Check sheet for the modelled part. Datum: model origin and axes. Units: mm. Face numbers are marked on the shaded views. A direction names the side the tool comes from. Round coordinates to 2 decimals unless told otherwise and drop trailing zeros. Loops run counter-clockwise (first coordinate to the right, second up) from the corner with the lowest first, then second, coordinate; pieces in that order, holes last. Notation, with made-up numbers: (51.5, 44.5) - (91.5, 44.5) arc R28 cw to (91.5, 73.5) - close; hole circle Ø8 at (29.5, 81.25). An arc over 180 degrees is marked (long way). Answer in a Markdown table with one row per item. Add a question column.
(1) Cross-section at D-D on y = 9.25. Enter the section's corners in (x, z) (3 decimals), then the cut area to 3 significant figures.
(2) Cross-section at B-B on x = 22. Enter the section's corners in (y, z), then the cut area to 3 significant figures.
(3) Thickness scan on line 1 along X through (y, z) = (-10, 9.5); line 2 along X through (y, z) = (6, 4); line 3 along Z through (x, y) = (25.4, 1.5) (3 decimals). Record the ranges inside material, lowest first.
(4) Access from +Z, -Z, +X, -X, +Y, -Y to the whole of each face (thin tool, end or side, straight path). Record for the marked faces 4, 5, 6, 7 and 8.
(5) Gauge pin test, flat ends, axial feed: pin 1 (1.1 mm diameter, centred on x = 14, y = 1, fed in from -Z); pin 2 (2 mm diameter, centred on y = 5, z = 18, fed in from +X); pin 3 (2 mm diameter, centred on x = 21, y = 4, fed in from +Z); pin 4 (7.5 mm diameter, centred on x = 25.4, z = 9.525, fed in from -Y). Record the tip position at first contact, or that the pin passes through.
(6) Cross-section at C-C on y = 3.75. Enter the section's corners in (x, z) (3 decimals).
(7) Mould release check, pull along X, two halves, no side actions. Record for the marked faces 1, 2 and 3: +X half, -X half, draft (parallel to the pull), parting line (faces both ways), or undercut.
(8) Cross-section at A-A on z = 7.5. Enter the section's corners in (x, y), then the cut area to 3 significant figures.
from build123d import *

# Parameters (mm, degrees)
F0_W     = 12.7
F0_H     = 25.4
F1_DEPTH = 12.7
F3_DEPTH = 12.7
F4_W     = 12.7
F4_H     = 12.7
F5_DEPTH = 12.7
F6_R     = 9.525
F7_DEPTH = 12.7
F8_R     = 6.35
F9_DEPTH = 25.4


with BuildPart() as f1:
    # F0 (on Front) → F1 (new body, symmetric)
    with BuildSketch(Plane.XZ):
        with Locations((6.35, 12.7)):
            Rectangle(F0_W, F0_H)
    extrude(amount=F1_DEPTH, both=True)

    # F2 (on face) → F3 (cut)
    with BuildSketch(Plane.YZ.offset(12.7)):
        Polygon((-12.7, 25.4), (-12.7, 19.05), (-6.35, 25.4), align=None)
        Polygon((12.7, 25.4), (6.35, 25.4), (12.7, 19.05), align=None)
    extrude(amount=-F3_DEPTH, mode=Mode.SUBTRACT)

    # F4 (on face) → F5 (join)
    with BuildSketch(Plane.YZ.offset(12.7)):
        with Locations((0, 12.7)):
            Rectangle(F4_W, F4_H)
    extrude(amount=F5_DEPTH)

    # F6 (on Front) → F7 (join, symmetric)
    with BuildSketch(Plane.XZ):
        with Locations((25.4, 9.525)):
            Circle(F6_R)
    extrude(amount=F7_DEPTH, both=True)

    # F8 (on face) → F9 (cut)
    with BuildSketch(Plane.XZ.offset(12.7)):
        with Locations((25.4, 9.525)):
            Circle(F8_R)
    extrude(amount=-F9_DEPTH, mode=Mode.SUBTRACT)


solid = f1.part
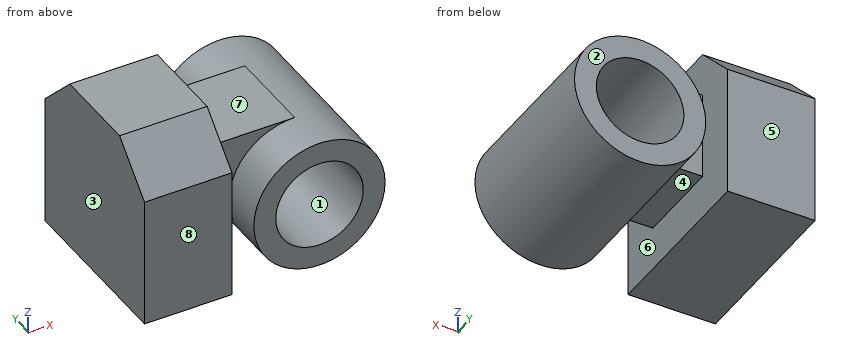
Answers:
| question | item | result |
|---|---|---|
| 1 | outline | (0, 0) - (12.7, 0) - (12.7, 22.5) - (0, 22.5) - close; circle Ø19.05 at (25.4, 9.525); hole circle Ø12.7 at (25.4, 9.525) |
| 1 | area | 444 mm^2 |
| 2 | outline | (-12.7, 0.63) - (12.7, 0.63) - (12.7, 4.16) - (-12.7, 4.16) - close; (-12.7, 14.89) - (12.7, 14.89) - (12.7, 18.42) - (6.35, 18.42) - (6.35, 19.05) - (-6.35, 19.05) - (-6.35, 18.42) - (-12.7, 18.42) - close |
| 2 | area | 188 mm^2 |
| 3 | line 1 | x = 0 to 12.7, 15.88 to 19.05, 31.75 to 34.92 |
| 3 | line 2 | x = 0 to 12.7, 17.64 to 22.27, 28.53 to 33.16 |
| 3 | line 3 | z = 0 to 3.175, 15.875 to 19.05 |
| 4 | face 4 | -Z, +Y, -Y |
| 4 | face 5 | +Z, -Z, +X, -X, +Y |
| 4 | face 6 | none |
| 4 | face 7 | +Z, +X, +Y, -Y |
| 4 | face 8 | +Z, -Z, +X, -X, -Y |
| 5 | pin 1 | stops at z = 6.35 |
| 5 | pin 2 | stops at x = 31.3 |
| 5 | pin 3 | stops at z = 19.05 |
| 5 | pin 4 | passes through |
| 6 | outline | (0, 0) - (12.7, 0) - (12.7, 6.35) - (16.42, 6.35) arc R9.525 ccw (long way) to (25.4, 19.05) - (12.7, 19.05) - (12.7, 25.4) - (0, 25.4) - close; hole circle Ø12.7 at (25.4, 9.525) |
| 7 | face 1 | undercut |
| 7 | face 2 | draft |
| 7 | face 3 | -X half |
| 8 | outline | (0, -12.7) - (12.7, -12.7) - (12.7, -6.35) - (16.09, -6.35) - (16.09, -12.7) - (19.38, -12.7) - (19.38, 12.7) - (16.09, 12.7) - (16.09, 6.35) - (12.7, 6.35) - (12.7, 12.7) - (0, 12.7) - close; (31.42, -12.7) - (34.71, -12.7) - (34.71, 12.7) - (31.42, 12.7) - close |
| 8 | area | 533 mm^2 |
